Geometry check sheet. Reference: the model listing, model coordinates, mm. Face numbers are marked on the shaded views. A direction names the side the tool comes from. Coordinates: 2 decimals unless noted, no trailing zeros. Loops run counter-clockwise (first coordinate to the right, second up) from the corner with the lowest first, then second, coordinate; pieces in that order, holes last. Notation, with made-up numbers: (-0.75, 34.25) -> (51.25, 34.25) arc R19 ccw to (51.25, 42.25) -> close; hole circle Ø4 at (76.5, 55). An arc over 180 degrees is marked (long way). Answer as a JSON object with one key per item and string values.
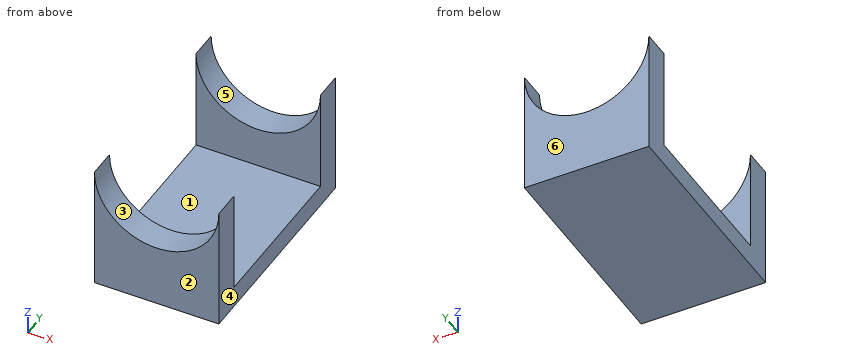
from build123d import *

# Parameters (mm, degrees)
SKETCH1_W           = 59.182
SKETCH1_H           = 59.182
BOSS_EXTRUDE2_DEPTH = 103.886
SKETCH4_R           = 29.591
CUT_EXTRUDE1_DEPTH  = 119.540559012
SKETCH6_W           = 59.182
SKETCH6_H           = 76.962
CUT_EXTRUDE2_DEPTH  = 129.342082086
SKETCH8_W           = 59.182
SKETCH8_H           = 10.20581791
BOSS_EXTRUDE3_DEPTH = 76.962


with BuildPart() as part:
    # Sketch1 → Boss-Extrude2 (new body)
    with BuildSketch(Plane(origin=(0, 0, 0), x_dir=(1, 0, 0), z_dir=(0, 1, 0))):
        with Locations((-17.066045707, -3.313152031)):
            Rectangle(SKETCH1_W, SKETCH1_H)
    extrude(amount=BOSS_EXTRUDE2_DEPTH)

    # Sketch4 → Cut-Extrude1 (cut, through all)
    with BuildSketch(Plane.XZ):
        with Locations((-17.066045707, 32.904152031)):
            Circle(SKETCH4_R)
    extrude(amount=-CUT_EXTRUDE1_DEPTH, mode=Mode.SUBTRACT)

    # Sketch6 → Cut-Extrude2 (cut, through all)
    with BuildSketch(Plane(origin=(0, 0, -26.277847969), x_dir=(-1, 0, 0), z_dir=(0, 0, -1))):
        with Locations((17.066045707, 51.943)):
            Rectangle(SKETCH6_W, SKETCH6_H)
    extrude(amount=-CUT_EXTRUDE2_DEPTH, mode=Mode.SUBTRACT)


with BuildPart() as cut_extrude2_piece_1:
    # of the separate pieces the step leaves, piece 1, a body of its own (cut_extrude2_pieces)
    add(part.part.solids().sort_by_distance((12.524954293, 90.424, -26.277847969))[0])



with BuildPart() as cut_extrude2_piece_2:
    # of the separate pieces the step leaves, piece 2, a body of its own (cut_extrude2_pieces)
    add(part.part.solids().sort_by_distance((-46.657045707, 0, -26.277847969))[0])


with BuildPart() as cut_extrude2_piece_1_1:
    add(cut_extrude2_piece_1.part)

    add(cut_extrude2_piece_2.part)  # Boss-Extrude3 merges Cut-Extrude2 piece 2
    # Sketch8 → Boss-Extrude3 (add)
    with BuildSketch(Plane.XZ.offset(-90.424)):
        with Locations((-17.066045707, -21.174939014)):
            Rectangle(SKETCH8_W, SKETCH8_H)
    extrude(amount=BOSS_EXTRUDE3_DEPTH)


solid = cut_extrude2_piece_1_1.part
1. Section check C-C, the plane x = -9. Record the boundary of the cut face in (y, z), then the cut area to 3 significant figures.
Evaluation:
{"outline": "(0, -26.28) -> (103.89, -26.28) -> (103.89, 4.43) -> (90.42, 4.43) -> (90.42, -16.07) -> (13.46, -16.07) -> (13.46, 4.43) -> (0, 4.43) -> close", "area": "1,610 mm^2"}
2. Mould release check, pull along X, two halves, no side actions. Record for the marked faces 3, 4, 5 and 6: released by +X, released by -X, zero draft, split by the parting line, or undercut.
Evaluation:
{"face 3": "undercut", "face 4": "released by +X", "face 5": "undercut", "face 6": "zero draft"}
3. Section check D-D, the plane y = 51. Record the boundary of the cut face in (x, z), then the cut area to 3 significant figures.
Evaluation:
{"outline": "(-46.66, -26.28) -> (12.52, -26.28) -> (12.52, -16.07) -> (-46.66, -16.07) -> close", "area": "604 mm^2"}
4. Tool access check on the marked faces 1 and 2. Record the directions out of +Z, -Z, +X, -X, +Y, -Y that give a thin tool (end or side, any length) a straight path to the whole face; none if there is none.
Evaluation:
{"face 1": "+Z, +X, -X", "face 2": "+Z, -Z, +X, -X, -Y"}
5. Section check B-B, the plane z = 27.5. Record the boundary of the cut face in (x, y).
Evaluation:
{"outline": "(-46.66, 0) -> (-46.16, 0) -> (-46.16, 13.46) -> (-46.66, 13.46) -> close; (-46.66, 90.42) -> (-46.16, 90.42) -> (-46.16, 103.89) -> (-46.66, 103.89) -> close; (12.03, 0) -> (12.52, 0) -> (12.52, 13.46) -> (12.03, 13.46) -> close; (12.03, 90.42) -> (12.52, 90.42) -> (12.52, 103.89) -> (12.03, 103.89) -> close"}
6. Thickness scan on probe 1 along Y at (x, z) = (-44, -14.5); probe 2 along Z at (x, y) = (3.5, 68.5); probe 3 along X at (y, z) = (90.5, 10). Record the ranges inside material, lowest first. Write a range as from..to.
Evaluation:
{"probe 1": "y = 0..13.46, 90.42..103.89", "probe 2": "z = -26.28..-16.07", "probe 3": "x = -46.66..-35.8, 1.67..12.52"}
7. Depth check by flat-ended pin: P1, Ø4, axis at x = -23, y = 77, coming from the +Z side. Enter the tip coordinate at first touch or a pass-through.
Evaluation:
{"P1": "stops at z = -16.07"}
8. Section check A-A, the plane z = -2. Record the boundary of the cut face in (x, y).
Evaluation:
{"outline": "(-46.66, 0) -> (12.52, 0) -> (12.52, 13.46) -> (-46.66, 13.46) -> close; (-46.66, 90.42) -> (12.52, 90.42) -> (12.52, 103.89) -> (-46.66, 103.89) -> close"}
